from build123d import *

# Parameters (mm, degrees)
SKETCH1_W             = 16
SKETCH1_H             = 16
FRONT_OF_SWITCH_DEPTH = 1.5
SKETCH2_W             = 16
SKETCH2_H             = 16
SKETCH2_W_2           = 14
SKETCH2_H_2           = 14
SIDES_OF_SWITCH_DEPTH = 3.5
SKETCH3_W             = 22
SKETCH3_H             = 22
SKETCH3_W_2           = 14
SKETCH3_H_2           = 14
BOSS_EXTRUDE3_DEPTH   = 2
SKETCH4_R             = 5.5
BOSS_EXTRUDE4_DEPTH   = 4
BOSS_EXTRUDE5_START   = -2
SKETCH5_R             = 5.5
SKETCH5_W             = 5.5
SKETCH5_H             = 5.5
BOSS_EXTRUDE5_DEPTH   = 2
SKETCH6_W             = 5.5
SKETCH6_H             = 5.5
BOSS_EXTRUDE6_DEPTH   = 1


with BuildPart() as part:
    # Sketch1 → Front of switch (new body)
    with BuildSketch(Plane.XY):
        Rectangle(SKETCH1_W, SKETCH1_H)
    extrude(amount=FRONT_OF_SWITCH_DEPTH)

    # Sketch2 → Sides of switch (add)
    with BuildSketch(Plane(origin=(0, 0, 0), x_dir=(-1, 0, 0), z_dir=(0, 0, -1))):
        Rectangle(SKETCH2_W, SKETCH2_H)
        Rectangle(SKETCH2_W_2, SKETCH2_H_2, mode=Mode.SUBTRACT)
    extrude(amount=SIDES_OF_SWITCH_DEPTH)

    # Sketch3 → Boss-Extrude3 (add)
    with BuildSketch(Plane(origin=(0, 0, -3.5), x_dir=(-1, 0, 0), z_dir=(0, 0, -1))):
        Rectangle(SKETCH3_W, SKETCH3_H)
        Rectangle(SKETCH3_W_2, SKETCH3_H_2, mode=Mode.SUBTRACT)
    extrude(amount=BOSS_EXTRUDE3_DEPTH)

    # Sketch4 → Boss-Extrude4 (add)
    with BuildSketch(Plane(origin=(0, 11, 0), x_dir=(1, 0, 0), z_dir=(0, 1, 0))):
        with BuildLine():
            Line((-8, 5.5), (-8, 11))
            ThreePointArc((-8, 11), (0, 19), (8, 11))
            Line((8, 11), (8, 5.5))
            Line((8, 5.5), (8, 3.5))
            Line((8, 3.5), (-8, 3.5))
            Line((-8, 3.5), (-8, 5.5))
        make_face()
        with Locations(Location((0, 11, 0), (0, 0, 270))):
            Circle(SKETCH4_R, mode=Mode.SUBTRACT)
    extrude(amount=-BOSS_EXTRUDE4_DEPTH)

    # Sketch5 → Boss-Extrude5 (add)
    with BuildSketch(Plane.XZ.offset(-7).offset(BOSS_EXTRUDE5_START)):
        with Locations(Location((0, -11, 0), (0, 0, 90))):
            Circle(SKETCH5_R)
        with Locations((0, -11)):
            Rectangle(SKETCH5_W, SKETCH5_H, mode=Mode.SUBTRACT)
    extrude(amount=BOSS_EXTRUDE5_DEPTH)

    # Sketch6 → Boss-Extrude6 (add)
    with BuildSketch(Plane.XZ.offset(-7)):
        with Locations((0, -11)):
            Rectangle(SKETCH6_W, SKETCH6_H)
    extrude(amount=-BOSS_EXTRUDE6_DEPTH)


solid = part.part
Here's how the part is built. I have some questions about the finished solid (model axes, mm). A direction names the side the tool comes from. Coordinates: 2 decimals unless noted, no trailing zeros. Write each loop counter-clockwise with the first axis right and the second up, starting at its lowest first coordinate (ties: lowest second). Pieces come first, ordered by that corner, then holes.
Item 1: If we mould it in two halves opening along Z, with no side actions, what happens to faces 1 (the flat face through (0, 9, -7)), 2 (the flat face through (0, 7, -9)), 3 (the cylindrical face through (0, 9, -19)), 4 (the flat face through (0, 8.5, -13.75))? For each: +Z half, -Z half, draft (parallel to the pull), parting line (faces both ways), or undercut.
Item 2: Will these pins go through, and if not, where does the flat tip stop? pin 1 (12 mm diameter, centred on y = 3, z = -13, fed in from -X); pin 2 (12 mm diameter, centred on x = 0, y = 2.5, fed in from -Z); pin 3 (6.5 mm diameter, centred on x = -4.5, y = -3.5, fed in from -Z); pin 4 (1.5 mm diameter, centred on x = -1, z = 0, fed in from -Y).
Item 3: I want a section at B-B on z = -2.5. Write out the boundary of the cut face in (x, y).
Item 4: On a 3-axis mill with a long thin cutter (end or side, diameter ignored), from which of +Z, -Z, +X, -X, +Y, -Y can I reach the whole of each face in a straight line? I mean faces 5 (the flat face through (-8, 0, -1)), 6 (the flat face through (2.75, 8.5, -11)), 7 (the flat face through (0, -7, -3)), 8 (the flat face through (8, 0, -1)). Say none if no direction works.
Item 5: If I drill on line 1 (X direction, y = 9.9, z = -11); line 2 (Z direction, x = 0, y = 9.9); line 3 (Y direction, x = -5.75, z = -3), over which ranges is the centre line in solid material (lowest first)?
Item 6: I want a section at D-D on x = 0. Write out the boundary of the cut face in (y, z), and give its area (3 significant figures).
Item 7: I want a section at C-C on y = 6. Write out the boundary of the cut face in (x, z), and give its area (3 significant figures).
Item 8: I want a section at A-A on y = 9.75. Write out the boundary of the cut face in (x, z), and give its area (3 significant figures).
Findings below:
1. face 1: undercut
1. face 2: draft
1. face 3: -Z half
1. face 4: undercut
2. pin 1: stops at x = -8
2. pin 2: stops at z = -19
2. pin 3: stops at z = -5.5
2. pin 4: stops at y = -8
3. outline: (-8, -8) - (8, -8) - (8, 8) - (-8, 8) - close; hole (-7, -7) - (7, -7) - (7, 7) - (-7, 7) - close
4. face 5: +Z, -X, +Y, -Y
4. face 6: +Y
4. face 7: -Z
4. face 8: +Z, +X, +Y, -Y
5. line 1: x = -8 to -5.5, 5.5 to 8
5. line 2: z = -19 to -16.5, -5.5 to -3.5
5. line 3: y = -8 to -7, 7 to 8
6. outline: (-11, -5.5) - (-7, -5.5) - (-7, 0) - (7, 0) - (7, -19) - (11, -19) - (11, -16.5) - (9, -16.5) - (9, -13.75) - (8, -13.75) - (8, -8.25) - (9, -8.25) - (9, -5.5) - (11, -5.5) - (11, -3.5) - (8, -3.5) - (8, 1.5) - (-8, 1.5) - (-8, -3.5) - (-11, -3.5) - close
6. area: 73.5 mm2
7. outline: (-11, -5.5) - (-7, -5.5) - (-7, 0) - (7, 0) - (7, -5.5) - (11, -5.5) - (11, -3.5) - (8, -3.5) - (8, 1.5) - (-8, 1.5) - (-8, -3.5) - (-11, -3.5) - close
7. area: 47.0 mm2
8. outline: (-11, -5.5) - (-8, -5.5) - (-8, -11) arc R8 ccw to (8, -11) - (8, -5.5) - (11, -5.5) - (11, -3.5) - (-11, -3.5) - close; hole circle Ø11 at (0, -11)
8. area: 137 mm2
